The listing builds one solid part. Answer for the finished solid, in the listing's coordinates (mm). Face numbers are marked on the shaded views. Give positions to 0.01 mm unless a question says otherwise; leave off trailing zeros. Order: outer loops, then holes, each group sorted by start corner. A loop starts at its lowest first (then second) coordinate and runs counter-clockwise, first axis right, second up. Notation, with made-up numbers: (74.25, 45.5) - (129.25, 45.5) arc R36 cw to (129.25, 80.5) - close; hole circle Ø11 at (-27, 84.25). An arc over 180 degrees is marked (long way). Use CSV: the item, a comma, the result in double quotes.
```python
from build123d import *

# Parameters (mm, degrees)
SKETCH_1_W          = 102
SKETCH_1_H          = 40
EXTRUDE_1_DEPTH     = 5
SKETCH_2_R          = 1.5
CUT_EXTRUDE_1_DEPTH = 56.009090158
SKETCH_3_R          = 2
CUT_EXTRUDE_2_DEPTH = 5
FILLET_1_R          = 8


with BuildPart() as part:
    # Sketch 1 → Extrude 1 (new body)
    with BuildSketch(Plane(origin=(0, 0, 0), x_dir=(1, 0, 0), z_dir=(0, 1, 0))):
        Rectangle(SKETCH_1_W, SKETCH_1_H)
    extrude(amount=EXTRUDE_1_DEPTH)

    # Sketch 2 → Cut-Extrude 1 (cut, through all)
    with BuildSketch(Plane(origin=(0, 5, 0), x_dir=(1, 0, 0), z_dir=(0, 1, 0))):
        with Locations(Location((-46, 3, 0), (0, 0, 270))):
            Circle(SKETCH_2_R)
        with Locations(Location((-28, 3, 0), (0, 0, 270))):
            Circle(SKETCH_2_R)
        with Locations(Location((-28, -3, 0), (0, 0, 270))):
            Circle(SKETCH_2_R)
        with Locations(Location((-46, -3, 0), (0, 0, 270))):
            Circle(SKETCH_2_R)
        with Locations(Location((-28, 15, 0), (0, 0, 270))):
            Circle(SKETCH_2_R)
        with Locations(Location((-28, 9, 0), (0, 0, 270))):
            Circle(SKETCH_2_R)
        with Locations(Location((-46, 15, 0), (0, 0, 270))):
            Circle(SKETCH_2_R)
        with Locations(Location((-46, 9, 0), (0, 0, 270))):
            Circle(SKETCH_2_R)
        with Locations(Location((-46, -9, 0), (0, 0, 270))):
            Circle(SKETCH_2_R)
        with Locations(Location((-46, -15, 0), (0, 0, 270))):
            Circle(SKETCH_2_R)
        with Locations(Location((-28, -9, 0), (0, 0, 270))):
            Circle(SKETCH_2_R)
        with Locations(Location((-28, -15, 0), (0, 0, 270))):
            Circle(SKETCH_2_R)
        with Locations(Location((28, -15, 0), (0, 0, 270))):
            Circle(SKETCH_2_R)
        with Locations(Location((28, -9, 0), (0, 0, 270))):
            Circle(SKETCH_2_R)
        with Locations(Location((46, -15, 0), (0, 0, 270))):
            Circle(SKETCH_2_R)
        with Locations(Location((46, -9, 0), (0, 0, 270))):
            Circle(SKETCH_2_R)
        with Locations(Location((46, 9, 0), (0, 0, 270))):
            Circle(SKETCH_2_R)
        with Locations(Location((46, 15, 0), (0, 0, 270))):
            Circle(SKETCH_2_R)
        with Locations(Location((28, 9, 0), (0, 0, 270))):
            Circle(SKETCH_2_R)
        with Locations(Location((28, 15, 0), (0, 0, 270))):
            Circle(SKETCH_2_R)
        with Locations(Location((46, -3, 0), (0, 0, 90))):
            Circle(SKETCH_2_R)
        with Locations(Location((28, -3, 0), (0, 0, 270))):
            Circle(SKETCH_2_R)
        with Locations(Location((28, 3, 0), (0, 0, 270))):
            Circle(SKETCH_2_R)
        with Locations(Location((46, 3, 0), (0, 0, 270))):
            Circle(SKETCH_2_R)
    extrude(amount=-CUT_EXTRUDE_1_DEPTH, mode=Mode.SUBTRACT)

    # Sketch 3 → Cut-Extrude 2 (cut)
    with BuildSketch(Plane(origin=(0, 5, 0), x_dir=(1, 0, 0), z_dir=(0, 1, 0))):
        with Locations(Location((-12.5, 10, 0), (0, 0, 270))):
            Circle(SKETCH_3_R)
        with Locations(Location((12.5, 10, 0), (0, 0, 270))):
            Circle(SKETCH_3_R)
        with Locations(Location((12.5, -10, 0), (0, 0, 270))):
            Circle(SKETCH_3_R)
        with Locations(Location((-12.5, -10, 0), (0, 0, 270))):
            Circle(SKETCH_3_R)
    extrude(amount=-CUT_EXTRUDE_2_DEPTH, mode=Mode.SUBTRACT)

    # Fillet 1
    fillet_1_edges = [part.edges().sort_by_distance(p)[0] for p in [
        (-51, 2.5, -20),
        (51, 2.5, -20),
        (51, 2.5, 20),
        (-51, 2.5, 20),
    ]]
    fillet(fillet_1_edges, radius=FILLET_1_R)


solid = part.part
```
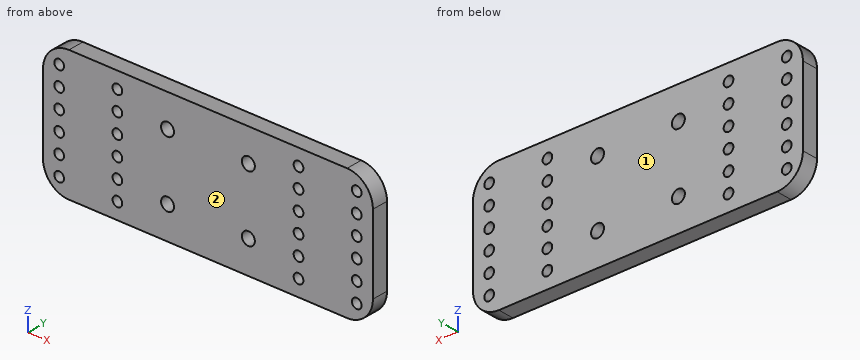
Item 1: The part is cut by section C-C (x = 46). Give the vertices of the cut face in (y, z), and give its area (3 significant figures).
Taken from the geometry:
outline,"(0, -19.42) - (5, -19.42) - (5, -16.5) - (0, -16.5) - close; (0, -13.5) - (5, -13.5) - (5, -10.5) - (0, -10.5) - close; (0, -7.5) - (5, -7.5) - (5, -4.5) - (0, -4.5) - close; (0, -1.5) - (5, -1.5) - (5, 1.5) - (0, 1.5) - close; (0, 4.5) - (5, 4.5) - (5, 7.5) - (0, 7.5) - close; (0, 10.5) - (5, 10.5) - (5, 13.5) - (0, 13.5) - close; (0, 16.5) - (5, 16.5) - (5, 19.42) - (0, 19.42) - close"
area,"104 mm^2"
Item 2: The part is cut by section B-B (z = -9). Give the vertices of the cut face in (x, y), and give its area (3 significant figures).
Taken from the geometry:
outline,"(-51, 0) - (-47.5, 0) - (-47.5, 5) - (-51, 5) - close; (-44.5, 0) - (-29.5, 0) - (-29.5, 5) - (-44.5, 5) - close; (-26.5, 0) - (-14.23, 0) - (-14.23, 5) - (-26.5, 5) - close; (-10.77, 0) - (10.77, 0) - (10.77, 5) - (-10.77, 5) - close; (14.23, 0) - (26.5, 0) - (26.5, 5) - (14.23, 5) - close; (29.5, 0) - (44.5, 0) - (44.5, 5) - (29.5, 5) - close; (47.5, 0) - (51, 0) - (51, 5) - (47.5, 5) - close"
area,"415 mm^2"
Item 3: The mould has two halves that part along Y. Classify the marked faces 1 and 2: +Y half, -Y half, draft (parallel to the pull), parting line (faces both ways), or undercut.
Taken from the geometry:
face 1,"+Y half"
face 2,"-Y half"
Item 4: This flat-tipped pin is pushed along its axis until it touches: pin 1 (3 mm diameter, centred on x = -12.5, z = -10, fed in from -Y). Where does it stop, or does it pass through?
Taken from the geometry:
pin 1,"through"
Item 5: Find the intervals of material crossed by line 1 along X through (y, z) = (3.1, 3); line 2 along Z through (x, y) = (-13, 2.65); line 3 along Z through (x, y) = (11.5, 4.75), in increasing order.
Taken from the geometry:
line 1,"-51 to -47.5, -44.5 to -29.5, -26.5 to 26.5, 29.5 to 44.5, 47.5 to 51"
line 2,"-20 to -11.94, -8.06 to 8.06, 11.94 to 20"
line 3,"-20 to -11.73, -8.27 to 8.27, 11.73 to 20"
Item 6: The part is cut by section D-D (z = 15). Give the vertices of the cut face in (x, y).
Taken from the geometry:
outline,"(-50.42, 0) - (-47.5, 0) - (-47.5, 5) - (-50.42, 5) - close; (-44.5, 0) - (-29.5, 0) - (-29.5, 5) - (-44.5, 5) - close; (-26.5, 0) - (26.5, 0) - (26.5, 5) - (-26.5, 5) - close; (29.5, 0) - (44.5, 0) - (44.5, 5) - (29.5, 5) - close; (47.5, 0) - (50.42, 0) - (50.42, 5) - (47.5, 5) - close"
Item 7: The part is cut by section A-A (x = 12.5). Give the vertices of the cut face in (y, z), and give its area (3 significant figures).
Taken from the geometry:
outline,"(0, -20) - (5, -20) - (5, -12) - (0, -12) - close; (0, -8) - (5, -8) - (5, 8) - (0, 8) - close; (0, 12) - (5, 12) - (5, 20) - (0, 20) - close"
area,"160 mm^2"
